Read the model definition and answer for the solid it produces. Units are mm, in the model's axes. A direction names the side the tool comes from. Give positions to 0.01 mm unless a question says otherwise; leave off trailing zeros. Write each loop counter-clockwise with the first axis right and the second up, starting at its lowest first coordinate (ties: lowest second). Pieces come first, ordered by that corner, then holes. Notation, with made-up numbers: M -28.5,-30 L 24.5,-30 A20 cw 24.5,1 Z; hole C 17.25,-39.5 d4. An arc over 180 degrees is marked long. Answer as CSV lines item,"result". Start each with the question number.
```python
from build123d import *

# Parameters (mm, degrees)
SKETCH1_R           = 11
BOSS_EXTRUDE1_DEPTH = 35
SHELL1_T            = -1
SKETCH4_W           = 4
SKETCH4_H           = 5
CUT_EXTRUDE1_DEPTH  = 56.018178814
CIRPATTERN1_COUNT   = 8
CUT_EXTRUDE2_REACH  = 40.301
SKETCH5_R           = 1.5


with BuildPart() as part:
    # Sketch1 → Boss-Extrude1 (new body)
    with BuildSketch(Plane(origin=(0, 0, 0), x_dir=(1, 0, 0), z_dir=(0, 1, 0))):
        with Locations(Location((0, 0, 0), (0, 0, 270))):
            Circle(SKETCH1_R)
    extrude(amount=BOSS_EXTRUDE1_DEPTH)

    # Shell1
    shell1_openings = [part.faces().sort_by_distance(p)[0] for p in [
        (0, 0, 0),
    ]]
    offset(amount=SHELL1_T, openings=shell1_openings, kind=Kind.INTERSECTION)

    # Sketch4 → Cut-Extrude1 (cut, symmetric)
    with BuildSketch(Plane(origin=(30, 0, 0), x_dir=(0, 0, -1), z_dir=(1, 0, 0))):
        with Locations((0, 2.5)):
            Rectangle(SKETCH4_W, SKETCH4_H)
    cut_extrude1 = extrude(amount=CUT_EXTRUDE1_DEPTH, both=True, mode=Mode.SUBTRACT)

    # CirPattern1: Cut-Extrude1 ×8 about axis
    cirpattern1_axis = Axis((0, 0, 0), (0, 1, 0))
    for i in range(1, CIRPATTERN1_COUNT):
        add(cut_extrude1.rotate(cirpattern1_axis, i * 360 / CIRPATTERN1_COUNT), mode=Mode.SUBTRACT)

    # Sketch5 → Cut-Extrude2 (cut, up to next)
    with BuildSketch(Plane(origin=(0, 35, 0), x_dir=(1, 0, 0), z_dir=(0, 1, 0)), mode=Mode.PRIVATE) as cut_extrude2_sk1:
        with Locations(Location((0, 0, 0), (0, 0, 270))):
            Circle(SKETCH5_R)
    cut_extrude2_tool1 = extrude(cut_extrude2_sk1.sketch, amount=-CUT_EXTRUDE2_REACH, mode=Mode.PRIVATE) & part.part
    add(cut_extrude2_tool1.solids().sort_by_distance((0, 35, 0))[0], mode=Mode.SUBTRACT)


solid = part.part
```
1. Find the intervals of material crossed by line 1 (X direction, y = 25, z = 0); line 2 (X direction, y = 34.85, z = 0), in increasing order. Write a range as [from, to].
2. Find section D-D on z = -3.75. Determine the outline of the cut face in (x, y), then the cut area to 3 significant figures.
3. Find section A-A on z = 0. Determine the outline of the cut face in (x, y).
4. Find section B-B on x = 0. Determine the outline of the cut face in (y, z), then the cut area to 3 significant figures.
5. Given pin 1 (1.3 mm diameter, centred on x = -1, z = 10.5, fed in from -Y); pin 2 (0.8 mm diameter, centred on x = -10.5, y = 3, fed in from +Z); pin 3 (6 mm diameter, centred on x = -6.5, y = 17.5, fed in from +Z), each flat-ended and moving along its own axis, determine where each tip first touches the part or whether it passes through.
6. Determine the mould class of faces 4 (the face through (10, 2, -2)), 5 (the face through (0, 34, 2)), 6 (the face through (-4, 0, 10)) for opening direction Z: +Z half, -Z half, draft (parallel to the pull), parting line (faces both ways), or undercut.
7. For faces 1 (the face through (4, 0, -10)), 2 (the face through (-2, 2, 10)), 3 (the face through (-10, 2, -2)), determine the directions among +Z, -Z, +X, -X, +Y, -Y from which every point of the face is accessible in a straight line to the end or side of a thin tool.
8. Find section C-C on y = 16.5. Determine the outline of the cut face in (x, z), then the cut area to 3 significant figures.
Computed:
1,line 1,"x = [-11, -10], [10, 11]"
1,line 2,"x = [-11, -1.5], [1.5, 11]"
2,outline,"M -10.34,0 L -9.27,0 L -9.27,34 L 9.27,34 L 9.27,0 L 10.34,0 L 10.34,35 L -10.34,35 Z"
2,area,"93.5 mm^2"
3,outline,"M -11,5 L -10,5 L -10,34 L -1.5,34 L -1.5,35 L -11,35 Z; M 1.5,34 L 10,34 L 10,5 L 11,5 L 11,35 L 1.5,35 Z"
4,outline,"M 5,-11 L 35,-11 L 35,-1.5 L 34,-1.5 L 34,-10 L 5,-10 Z; M 5,10 L 34,10 L 34,1.5 L 35,1.5 L 35,11 L 5,11 Z"
4,area,"77.0 mm^2"
5,pin 1,"stops at y = 5"
5,pin 2,"stops at z = 4.36"
5,pin 3,"stops at z = 10.43"
6,face 4,"undercut"
6,face 5,"undercut"
6,face 6,"draft"
7,face 1,"+Z, -Z, +X, -X, -Y"
7,face 2,"+Z, -Z, -Y"
7,face 3,"+X, -X, -Y"
8,outline,"C 0,0 d22; hole C 0,0 d20"
8,area,"66.0 mm^2"
